Check sheet for the modelled part. Datum: model origin and axes. Units: mm. A direction names the side the tool comes from. Coordinates: 2 decimals unless noted, no trailing zeros. Loops run counter-clockwise (first coordinate to the right, second up) from the corner with the lowest first, then second, coordinate; pieces in that order, holes last. Notation, with made-up numbers: (26, -28.75) - (39, -28.75) arc R30 cw to (39, 1.25) - close; hole circle Ø1 at (69, 79.25). An arc over 180 degrees is marked (long way). Write each question's results on one line, items separated by ' | '. Start each with the question number.
1. Cross-section at A-A (y = 0). Record the cut outline in (x, z).
2. Tool access check on faces 4 (the face through (4.517, 0, -61)), 5 (the face through (2.603, 0.02, -60.757)), 6 (the face through (8, 12.7, -61)). Record the directions out of +Z, -Z, +X, -X, +Y, -Y that give a thin tool (end or side, any length) a straight path to the whole face; none if there is none.
3. Gauge pin test, flat ends, axial feed: P1, Ø10, axis at x = -1, y = -6.5, coming from the +Z side; P2, Ø1.6, axis at y = 0, z = -35, coming from the +X side; P3, Ø1.6, axis at x = -0.5, z = -98, coming from the +Y side. Record the tip position at first contact, or that the pin passes through.
4. Cross-section at B-B (z = -20.5). Give the number of separate pieces and of enclosed holes in the cut face, and give its area (3 significant figures).
5. Thickness scan on line 1 (X direction, y = 0, z = -80); line 2 (X direction, y = -2, z = 3); line 3 (X direction, y = 9.5, z = -101.5). Record the ranges inside material, lowest first. Write a range as [from, to].
6. Draft check along X on faces 1 (the face through (12.7, 7, -61)), 2 (the face through (5.48, -7.04, -60.76)), 3 (the face through (-8, -12.7, -61)). Enter one of: released by +X, released by -X, zero draft, split by the parting line, or undercut.
```python
from build123d import *

# Parameters (mm, degrees)
BOSS_EXTRUDE1_DEPTH = 149


with BuildPart() as part:
    # Sketch1 → Boss-Extrude1 (new body)
    with BuildSketch(Plane.XY.offset(12.7)):
        with BuildLine():
            Line((-12.7, 10.5918), (-12.7, -10.5918))
            ThreePointArc((-12.7, -10.5918), (-12.082522516, -12.082522516), (-10.5918, -12.7))
            Line((-10.5918, -12.7), (-4.3561, -12.7))
            ThreePointArc((-4.3561, -12.7), (-3.2512, -11.5951), (-4.3561, -10.4902))
            Line((-4.3561, -10.4902), (-6.370083784, -10.4902))
            ThreePointArc((-6.370083784, -10.4902), (-7.34885674, -9.836204819), (-7.119204173, -8.681663397))
            Line((-7.119204173, -8.681663397), (-3.884643888, -5.447103113))
            ThreePointArc((-3.884643888, -5.447103113), (-2.854599756, -4.758849627), (-1.639579858, -4.517167143))
            Line((-1.639579858, -4.517167143), (1.639579858, -4.517167143))
            ThreePointArc((1.639579858, -4.517167143), (2.854599756, -4.758849627), (3.884643888, -5.447103113))
            Line((3.884643888, -5.447103113), (7.119204173, -8.681663397))
            ThreePointArc((7.119204173, -8.681663397), (7.34885674, -9.836204819), (6.370083784, -10.4902))
            Line((6.370083784, -10.4902), (4.356099789, -10.4902))
            ThreePointArc((4.356099789, -10.4902), (3.251199789, -11.5951), (4.356099789, -12.7))
            Line((4.356099789, -12.7), (10.5918, -12.7))
            ThreePointArc((10.5918, -12.7), (12.082522516, -12.082522516), (12.7, -10.5918))
            Line((12.7, -10.5918), (12.7, -4.3561))
            ThreePointArc((12.7, -4.3561), (11.5951, -3.2512), (10.4902, -4.3561))
            Line((10.4902, -4.3561), (10.4902, -6.370083784))
            ThreePointArc((10.4902, -6.370083784), (9.836204819, -7.34885674), (8.681663397, -7.119204173))
            Line((8.681663397, -7.119204173), (5.447103113, -3.884643888))
            ThreePointArc((5.447103113, -3.884643888), (4.758849627, -2.854599756), (4.517167143, -1.639579858))
            Line((4.517167143, -1.639579858), (4.517167143, 1.639579858))
            ThreePointArc((4.517167143, 1.639579858), (4.758849627, 2.854599756), (5.447103113, 3.884643888))
            Line((5.447103113, 3.884643888), (8.681663397, 7.119204173))
            ThreePointArc((8.681663397, 7.119204173), (9.836204819, 7.34885674), (10.4902, 6.370083784))
            Line((10.4902, 6.370083784), (10.4902, 4.3561))
            ThreePointArc((10.4902, 4.3561), (11.5951, 3.2512), (12.7, 4.3561))
            Line((12.7, 4.3561), (12.7, 10.5918))
            ThreePointArc((12.7, 10.5918), (12.082522516, 12.082522516), (10.5918, 12.7))
            Line((10.5918, 12.7), (4.3561, 12.7))
            ThreePointArc((4.3561, 12.7), (3.2512, 11.5951), (4.3561, 10.4902))
            Line((4.3561, 10.4902), (6.370083784, 10.4902))
            ThreePointArc((6.370083784, 10.4902), (7.34885674, 9.836204819), (7.119204173, 8.681663397))
            Line((7.119204173, 8.681663397), (3.884643888, 5.447103113))
            ThreePointArc((3.884643888, 5.447103113), (2.854599756, 4.758849627), (1.639579858, 4.517167143))
            Line((1.639579858, 4.517167143), (-1.639579858, 4.517167143))
            ThreePointArc((-1.639579858, 4.517167143), (-2.854599756, 4.758849627), (-3.884643888, 5.447103113))
            Line((-3.884643888, 5.447103113), (-7.119204173, 8.681663397))
            ThreePointArc((-7.119204173, 8.681663397), (-7.34885674, 9.836204819), (-6.370083784, 10.4902))
            Line((-6.370083784, 10.4902), (-4.356099789, 10.4902))
            ThreePointArc((-4.356099789, 10.4902), (-3.251199789, 11.5951), (-4.356099789, 12.7))
            Line((-4.356099789, 12.7), (-10.5918, 12.7))
            ThreePointArc((-10.5918, 12.7), (-12.082522516, 12.082522516), (-12.7, 10.5918))
        make_face()
        with BuildLine():
            Line((-8.681663397, 7.119204173), (-5.447103113, 3.884643888))
            ThreePointArc((-5.447103113, 3.884643888), (-4.758849627, 2.854599756), (-4.517167143, 1.639579858))
            Line((-4.517167143, 1.639579858), (-4.517167143, -1.639579858))
            ThreePointArc((-4.517167143, -1.639579858), (-4.758849627, -2.854599756), (-5.447103113, -3.884643888))
            Line((-5.447103113, -3.884643888), (-8.681663397, -7.119204173))
            ThreePointArc((-8.681663397, -7.119204173), (-9.836204819, -7.34885674), (-10.4902, -6.370083784))
            Line((-10.4902, -6.370083784), (-10.4902, 6.370083784))
            ThreePointArc((-10.4902, 6.370083784), (-9.836204819, 7.34885674), (-8.681663397, 7.119204173))
        make_face(mode=Mode.SUBTRACT)
        with BuildLine():
            ThreePointArc((-2.231856261, 1.340533427), (-2.28996531, 2.28996531), (-1.340533427, 2.231856261))
            ThreePointArc((-1.340533427, 2.231856261), (-1.1e-08, 2.603499998), (1.340533408, 2.231856273))
            ThreePointArc((1.340533408, 2.231856273), (2.28996531, 2.28996533), (2.231856262, 1.340533427))
            ThreePointArc((2.231856262, 1.340533427), (2.603499999, 1.1e-08), (2.231856274, -1.340533408))
            ThreePointArc((2.231856274, -1.340533408), (2.289965331, -2.28996531), (1.340533428, -2.231856262))
            ThreePointArc((1.340533428, -2.231856262), (6e-09, -2.603499999), (-1.340533417, -2.231856268))
            ThreePointArc((-1.340533417, -2.231856268), (-2.28996532, -2.28996532), (-2.231856267, -1.340533417))
            ThreePointArc((-2.231856267, -1.340533417), (-2.603499998, 6e-09), (-2.231856261, 1.340533427))
        make_face(mode=Mode.SUBTRACT)
    extrude(amount=-BOSS_EXTRUDE1_DEPTH)


solid = part.part
```
Established:
1) outline: (-12.7, -136.3) - (-10.49, -136.3) - (-10.49, 12.7) - (-12.7, 12.7) - close; (-4.52, -136.3) - (-2.6, -136.3) - (-2.6, 12.7) - (-4.52, 12.7) - close; (2.6, -136.3) - (4.52, -136.3) - (4.52, 12.7) - (2.6, 12.7) - close
2) face 4: +Z, -Z, +X | face 5: +Z, -Z | face 6: +Z, -Z, +X, -X, +Y
3) P1: z = 12.7 | P2: x = 4.52 | P3: y = 4.52
4) separate pieces: 1 | enclosed holes: 2 | area: 300 mm^2
5) line 1: [-12.7, -10.49], [-4.52, -2.6], [2.6, 4.52] | line 2: [-12.7, -10.49], [-4.54, -2.46], [2.46, 4.54] | line 3: [-12.7, -7.43], [7.43, 12.7]
6) face 1: released by +X | face 2: undercut | face 3: zero draft
